Geometry: final body of the model. Coordinates: model frame, mm. A direction names the side the tool comes from. Coordinates: 2 decimals unless noted, no trailing zeros. Loops run counter-clockwise (first coordinate to the right, second up) from the corner with the lowest first, then second, coordinate; pieces in that order, holes last. Notation, with made-up numbers: (72.5, -3.5) - (110.5, -3.5) arc R18 cw to (110.5, 31.5) - close; hole circle Ø3 at (42, 61.25). An arc over 180 degrees is marked (long way). Answer in a Markdown table with one row per item.
from build123d import *

# Parameters (mm, degrees)
SKETCH1_R                 = 5
BOSS_EXTRUDE1_DEPTH       = 10
BOSS_EXTRUDE3_DEPTH       = 2.4
SKETCH15_W                = 6.028380363
SKETCH15_H                = 2.991132054
CUT_EXTRUDE1_DEPTH        = 2.4
SKETCH16_W                = 6.590795167
SKETCH16_H                = 1.091372194
CUT_EXTRUDE3_DEPTH        = 2.4
M4X0_7_TAPPED_HOLE1_D     = 3.3
M4X0_7_TAPPED_HOLE1_DEPTH = 10.1
M4X0_7_TAPPED_HOLE1_TIP   = 0.991420021


with BuildPart() as part:
    # Sketch1 → Boss-Extrude1 (new body)
    with BuildSketch(Plane.XY):
        with Locations((-22.664426825, -3.702604382)):
            Circle(SKETCH1_R)
    extrude(amount=BOSS_EXTRUDE1_DEPTH)

    # Sketch2 → Boss-Extrude3 (add)
    with BuildSketch(Plane(origin=(0, 0, 0), x_dir=(-1, 0, 0), z_dir=(0, 0, -1))):
        with BuildLine():
            Line((25.526244429, -9.202604382), (19.80260922, -9.202604382))
            ThreePointArc((19.80260922, -9.202604382), (16.464426825, -3.702604382), (19.80260922, 1.797395618))
            Line((19.80260922, 1.797395618), (25.526244429, 1.797395618))
            ThreePointArc((25.526244429, 1.797395618), (28.864426825, -3.702604382), (25.526244429, -9.202604382))
        make_face()
    extrude(amount=BOSS_EXTRUDE3_DEPTH)

    # Sketch13 → Revolve1 (revolve)
    with BuildSketch(Plane(origin=(0, -3.702604382, 0), x_dir=(1, 0, 0), z_dir=(0, 1, 0)), mode=Mode.PRIVATE) as revolve1_sk:
        Polygon((-16.464426825, 2.4), (-22.664426825, 2.4), (-22.664426825, 8.6), align=None)
    revolve(revolve1_sk.sketch.rotate(Axis((-22.664426825, -3.702604382, -2.4), (0, 0, -1)), 180), axis=Axis((-22.664426825, -3.702604382, -2.4), (0, 0, -1)))

    # Sketch15 → Cut-Extrude1 (cut)
    with BuildSketch(Plane.XY.offset(-2.4)):
        with Locations((-22.512054248, 3.292961645)):
            Rectangle(SKETCH15_W, SKETCH15_H)
    extrude(amount=-CUT_EXTRUDE1_DEPTH, mode=Mode.SUBTRACT)

    # Sketch16 → Cut-Extrude3 (cut)
    with BuildSketch(Plane.XY.offset(-2.4)):
        with Locations((-23.098006803, -9.748290479)):
            Rectangle(SKETCH16_W, SKETCH16_H)
    extrude(amount=-CUT_EXTRUDE3_DEPTH, mode=Mode.SUBTRACT)

    # M4x0.7 Tapped Hole1
    with Locations(Plane.XY.offset(10)):
        with Locations((-22.664426825, -3.702604382)):
            Hole(M4X0_7_TAPPED_HOLE1_D / 2, depth=M4X0_7_TAPPED_HOLE1_DEPTH)
            with Locations((0, 0, -(M4X0_7_TAPPED_HOLE1_DEPTH + M4X0_7_TAPPED_HOLE1_TIP / 2))):  # 118° drill point
                Cone(0, M4X0_7_TAPPED_HOLE1_D / 2, M4X0_7_TAPPED_HOLE1_TIP, mode=Mode.SUBTRACT)


solid = part.part
(1) Cut plane B-B on z = 6. Output: boundary loops of the cut face in (x, y).
Verdict:
| item | result |
|---|---|
| outline | circle Ø10 at (-22.66, -3.7); hole circle Ø3.3 at (-22.66, -3.7) |
(2) First-contact query: pin 1 Ø5 at (x, z) = (-24, -6.5) entering from +Y; pin 2 Ø2 at (y, z) = (-4, 1.5) entering from +X; pin 3 Ø1 at (x, y) = (-23, -6.5) entering from -Z. Flat tips, straight axial feed; report the tip coordinate or a pass-through.
Verdict:
| item | result |
|---|---|
| pin 1 | stops at y = 0.77 |
| pin 2 | stops at x = -17.66 |
| pin 3 | stops at z = -6.28 |
(3) Access query for faces 1 (the face through (-17.895, -2.201, 4.93)), 2 (the face through (-23, 1.797, -2)). Directions: +Z, -Z, +X, -X, +Y, -Y. A direction counts if a zero-diameter tool reaches every point of the face in a straight line with its end or side. Return the directions, or none.
Verdict:
| item | result |
|---|---|
| face 1 | +Z |
| face 2 | +Z, -Z, +X, -X, +Y |
(4) Pull-direction query (X, two-part tool) for faces 3 (the face through (-22.4, -3.81, -0.92)), 4 (the face through (-23, -9.203, -2)), 5 (the face through (-16.465, -3.797, -1.183)); classes: pulls with the +X half, pulls with the -X half, needs draft (parallel to the pull), parting line crosses it, or undercut.
Verdict:
| item | result |
|---|---|
| face 3 | undercut |
| face 4 | needs draft |
| face 5 | pulls with the +X half |
(5) Cut plane A-A on z = -6. Output: boundary loops of the cut face in (x, y).
Verdict:
| item | result |
|---|---|
| outline | circle Ø5.2 at (-22.66, -3.7) |
(6) Ray query, probe 1 along X at (y, z) = (-3.75, 7); probe 2 along X at (y, z) = (-3, 0.5); probe 3 along Z at (x, y) = (-21, 1.25). Return the intervals inside material, ascending.
Verdict:
| item | result |
|---|---|
| probe 1 | x = -27.66 to -24.31, -21.02 to -17.66 |
| probe 2 | x = -27.61 to -24.16, -21.17 to -17.71 |
| probe 3 | z = -3.38 to 0 |
